```python
from build123d import *

# Parameters (mm, degrees)
PAD_DEPTH    = 8
SKETCH001_R  = 2.4
PAD001_DEPTH = 6


with BuildPart() as part:
    # Sketch → Pad (new body, symmetric)
    with BuildSketch(Plane.XY):
        with BuildLine():
            ThreePointArc((-2.5, 2.5), (-5, 0), (-2.5, -2.5))
            Line((-2.5, -2.5), (2.5, -2.5))
            ThreePointArc((2.5, -2.5), (5, 0), (2.5, 2.5))
            Line((2.5, 2.5), (-2.5, 2.5))
        make_face()
    extrude(amount=PAD_DEPTH, both=True)

    # Sketch001 (on Face5 of Pad) → Pad001 (join)
    with BuildSketch(Plane(origin=(0, 0, -8), x_dir=(1, 0, 0), z_dir=(0, 0, -1))):
        Circle(SKETCH001_R)
    extrude(amount=PAD001_DEPTH)


solid = part.part
```
Model file for the job. Use its own axes, mm. A direction names the side the tool comes from. Coordinates: 2 decimals unless noted, no trailing zeros. Loops run counter-clockwise (first coordinate to the right, second up) from the corner with the lowest first, then second, coordinate; pieces in that order, holes last. Notation, with made-up numbers: (-22.75, 34.5) - (16.25, 34.5) arc R14 ccw to (16.25, 58.5) - close; hole circle Ø4 at (-15.75, 47). An arc over 180 degrees is marked (long way). Write item = value, one per line. Start each with the question number.
Item 1: Saw through at A-A, the plane y = 0. List the corners of the cut face in (x, z), then the cut area to 3 significant figures.
Item 2: Wall check: probe 1 along Z at (x, y) = (-3.5, 1.9); probe 2 along X at (y, z) = (-0.35, 4.25); probe 3 along X at (y, z) = (-0.95, 5.5). Give the ranges that are in metal, low to high. Write a range as [from, to].
Item 3: Drop flat-ended pins along their axis: pin 1 Ø3 at (y, z) = (0.5, 3) entering from +X; pin 2 Ø2 at (x, y) = (4, -0.5) entering from -Z. Give the stop position or say it passes through.
Item 4: Saw through at D-D, the plane z = -1.5. List the corners of the cut face in (x, y).
Item 5: 3-axis set-ups, long thin cutter, end or side, ignore diameter. For faces 1 (the face through (1.29, -2.024, -10.958)), 2 (the face through (5, 0, 0)): which of +Z, -Z, +X, -X, +Y, -Y reach the whole face in a straight line?
Item 6: Saw through at B-B, the plane z = -8.5. List the corners of the cut face in (x, y), then the cut area to 3 significant figures.
Item 7: Saw through at C-C, the plane x = -0.5. List the corners of the cut face in (y, z), then the cut area to 3 significant figures.
Answers:
q1.outline = (-5, -8) - (-2.4, -8) - (-2.4, -14) - (2.4, -14) - (2.4, -8) - (5, -8) - (5, 8) - (-5, 8) - close
q1.area = 189 mm2
q2.probe_1 = [-8, 8]
q2.probe_2 = [-4.98, 4.98]
q2.probe_3 = [-4.81, 4.81]
q3.pin_1 = 5
q3.pin_2 = -8
q4.outline = (-2.5, -2.5) - (2.5, -2.5) arc R2.5 ccw to (2.5, 2.5) - (-2.5, 2.5) arc R2.5 ccw to start
q5.face_1 = -Z
q5.face_2 = +Z, -Z, +X
q6.outline = circle Ø4.8 at (0, 0)
q6.area = 18.1 mm2
q7.outline = (-2.5, -8) - (-2.35, -8) - (-2.35, -14) - (2.35, -14) - (2.35, -8) - (2.5, -8) - (2.5, 8) - (-2.5, 8) - close
q7.area = 108 mm2
